```python
from build123d import *

# Parameters (mm, degrees)
F1_DEPTH = 50


with BuildPart() as f1:
    # F0 (on Front) → F1 (new body)
    with BuildSketch(Plane.XZ):
        with BuildLine():
            Line((-4.419141, 8.010539), (-20.509183, 24.100582))
            Line((-20.509183, 24.100582), (-20.509183, -25.899418))
            Line((-20.509183, -25.899418), (-4.419141, -9.809375))
            ThreePointArc((-4.419141, -9.809375), (-8.109766, -0.899418), (-4.419141, 8.010539))
        make_face()
        with BuildLine():
            Line((29.490817, 24.100582), (-20.509183, 24.100582))
            Line((-20.509183, 24.100582), (-4.419141, 8.010539))
            ThreePointArc((-4.419141, 8.010539), (4.490817, 11.701165), (13.400774, 8.010539))
            Line((13.400774, 8.010539), (29.490817, 24.100582))
        make_face()
        with BuildLine():
            Line((-4.419141, -9.809375), (-20.509183, -25.899418))
            Line((-20.509183, -25.899418), (29.490817, -25.899418))
            Line((29.490817, -25.899418), (13.400774, -9.809375))
            ThreePointArc((13.400774, -9.809375), (4.490817, -13.5), (-4.419141, -9.809375))
        make_face()
        with BuildLine():
            Line((29.490817, -25.899418), (29.490817, 24.100582))
            Line((29.490817, 24.100582), (13.400774, 8.010539))
            ThreePointArc((13.400774, 8.010539), (16.132237, 3.922616), (17.091399, -0.899418))
            ThreePointArc((17.091399, -0.899418), (16.132237, -5.721452), (13.400774, -9.809375))
            Line((13.400774, -9.809375), (29.490817, -25.899418))
        make_face()
    extrude(amount=F1_DEPTH)


solid = f1.part
```
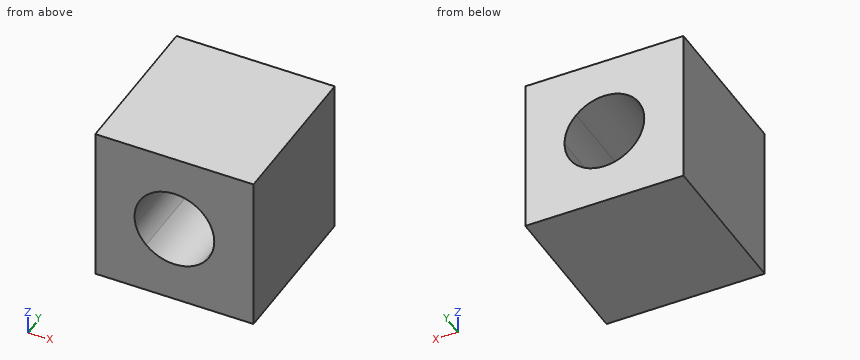
The model under review builds one solid part; all positions refer to its coordinate system, in mm. Give positions to 0.01 mm unless a question says otherwise; leave off trailing zeros. Order: outer loops, then holes, each group sorted by start corner. A loop starts at its lowest first (then second) coordinate and runs counter-clockwise, first axis right, second up. Notation, with made-up numbers: (18.5, -33) - (23.5, -33) arc R28 cw to (23.5, 0) - close; hole circle Ø4 at (84.25, -40). An arc over 180 degrees is marked (long way). Use CSV: the item, a comma, the result in double quotes. Start each with the question number.
Q1. We need section A-A, the plane x = -2.5. Write out the cut boundary in (y, z).
Q2. We need section B-B, the plane y = -46. Write out the cut boundary in (x, z).
Q3. We need section C-C, the plane z = -8. Write out the cut boundary in (x, y), and give its area (3 significant figures).
Q4. To check wall thickness, follow line 1 along X through (y, z) = (-8, -1); line 2 along Z through (x, y) = (-6.5, -31); line 3 along X through (y, z) = (-12, 8). State the ranges of each line that lie inside material, in increasing order. Write a range as [from, to].
Outcome:
1,outline,"(-50, -25.9) - (0, -25.9) - (0, -11.38) - (-50, -11.38) - close; (-50, 9.58) - (0, 9.58) - (0, 24.1) - (-50, 24.1) - close"
2,outline,"(-20.51, -25.9) - (29.49, -25.9) - (29.49, 24.1) - (-20.51, 24.1) - close; hole (-4.42, -9.81) arc R12.6 ccw to (13.4, -9.81) arc R12.6 ccw to (17.09, -0.9) arc R12.6 ccw to (13.4, 8.01) arc R12.6 ccw to (-4.42, 8.01) arc R12.6 ccw to start"
3,outline,"(-20.51, -50) - (-5.92, -50) - (-5.92, 0) - (-20.51, 0) - close; (14.9, -50) - (29.49, -50) - (29.49, 0) - (14.9, 0) - close"
3,area,"1,460 mm^2"
4,line 1,"x = [-20.51, -8.11], [17.09, 29.49]"
4,line 2,"z = [-25.9, -7.06], [5.26, 24.1]"
4,line 3,"x = [-20.51, -4.43], [13.41, 29.49]"
